```python
from build123d import *

# Parameters (mm, degrees)
SKETCH1_R             = 1.5500000000000012
BOSS_EXTRUDE1_DEPTH   = 1.5
SKETCH1_W             = 4.999999999999998
SKETCH1_H             = 10.5
BOSS_EXTRUDE1_2_DEPTH = 1.5
BOSS_EXTRUDE2_REACH   = 28.292
SKETCH2_R             = 2.500000000000001
SKETCH2_R_2           = 1.45
CUT_EXTRUDE1_DEPTH    = 25
FILLET1_R             = 2.5


with BuildPart() as part:
    # Sketch1 → Boss-Extrude1 (new, symmetric)
    with BuildSketch(Plane.XY):
        Polygon((-12.499999999999993, -2.4999999999999996), (-7.499999999999993, -2.5), (-7.499999999999993, 8), (-12.499999999999993, 8), align=None)
        with Locations((-9.999999999999995, 0)):
            Circle(SKETCH1_R, mode=Mode.SUBTRACT)
    extrude(amount=BOSS_EXTRUDE1_DEPTH, both=True)


with BuildPart() as body_2:
    # Sketch1 → Boss-Extrude1 2 (new, symmetric)
    with BuildSketch(Plane.XY):
        with Locations((10.000000000000007, 2.75)):
            Rectangle(SKETCH1_W, SKETCH1_H)
        with Locations((10.000000000000009, 2.45e-15)):
            Circle(SKETCH1_R, mode=Mode.SUBTRACT)
    extrude(amount=BOSS_EXTRUDE1_2_DEPTH, both=True)

    # Boss-Extrude2: up to this face of the body (flat: up to its plane)
    boss_extrude2_end = Plane(body_2.part.faces().sort_by_distance((12.5, 2.75, 0))[0])
    # Sketch2 → Boss-Extrude2 (add, up to the picked face)
    with BuildSketch(Plane.ZY.offset(12.499999999999993), mode=Mode.PRIVATE) as boss_extrude2_sk1:
        with Locations(Location((0, 8, 0), (0, 0, 306.869897646))):
            Circle(SKETCH2_R)
        with Locations((0, 8)):
            Circle(SKETCH2_R_2, mode=Mode.SUBTRACT)
    boss_extrude2_tool1 = split(extrude(boss_extrude2_sk1.sketch, amount=-BOSS_EXTRUDE2_REACH, mode=Mode.PRIVATE), bisect_by=boss_extrude2_end, keep=Keep.BOTH, mode=Mode.PRIVATE)

    add(part.part)  # Boss-Extrude2 merges part
    add(boss_extrude2_tool1.solids().sort_by(Axis((-12.5, 9.943431, -1.457574), (1, 0, 0)))[0])

    # Sketch2<2> → Cut-Extrude1 (cut)
    with BuildSketch(Plane.ZY.offset(12.499999999999993)):
        with BuildLine():
            Line((-1.4500000000000002, 8), (1.45, 8))
            ThreePointArc((1.45, 8), (9e-17, 9.45), (-1.45, 8))
        make_face()
        with BuildLine():
            ThreePointArc((-1.45, 8), (-2.7e-16, 6.55), (1.45, 8))
            Line((1.45, 8), (-1.4500000000000002, 8))
        make_face()
    extrude(amount=-CUT_EXTRUDE1_DEPTH, mode=Mode.SUBTRACT)

    # Fillet1
    fillet1_edges = [body_2.edges().sort_by_distance(p)[0] for p in [
        (7.500000000000007, -2.5, 0),
        (-7.499999999999993, -2.5, 0),
        (-12.499999999999993, -2.4999999999999996, 0),
        (12.500000000000007, -2.5, 0),
    ]]
    fillet(fillet1_edges, radius=FILLET1_R - 0.0001)  # a hair under: the kernel refuses the full size


solid = body_2.part
```
Check sheet for the modelled part. Datum: model origin and axes. Units: mm. A direction names the side the tool comes from. Give positions to 0.01 mm unless a question says otherwise; leave off trailing zeros. Order: outer loops, then holes, each group sorted by start corner. A loop starts at its lowest first (then second) coordinate and runs counter-clockwise, first axis right, second up. Notation, with made-up numbers: M 31.5,-5.75 L 49.5,-5.75 A29 cw 49.5,15.25 Z; hole C -21,18.5 d5. An arc over 180 degrees is marked long. Answer in a Markdown table with one row per item.
1) Cross-section at C-C, the plane x = -9.25. Enter the section's corners in (y, z), plus the area to 3 significant figures.
Filled sheet:
| item | result |
|---|---|
| outline | M -2.38,-1.5 L -1.36,-1.5 L -1.36,1.5 L -2.38,1.5 Z; M 1.36,-1.5 L 6,-1.5 A2.5 ccw long 6,1.5 L 1.36,1.5 Z; hole C 8,0 d2.9 |
| area | 29.0 mm2 |
2) Access from +Z, -Z, +X, -X, +Y, -Y to the whole of each face (thin tool, end or side, straight path). Record for faces 1 (the cylindrical face through (-0.175, 10.488, 0.246)), 2 (the cylindrical face through (8.213, -1.748, 0.021)), 3 (the flat face through (10, 3, -1.5)), 4 (the cylindrical face through (-11.14, 1.05, -0.02)), 5 (the flat face through (10, 3, 1.5)).
Filled sheet:
| item | result |
|---|---|
| face 1 | none |
| face 2 | +Z, -Z, -Y |
| face 3 | -Z, +X, -X, -Y |
| face 4 | +Z, -Z |
| face 5 | +Z, +X, -X, -Y |
3) Thickness scan on L1, parallel to Z at x = -1.5, y = 8; L2, parallel to Y at x = 10, z = -0.85; L3, parallel to Y at x = 11, z = -0.5. Record the ranges inside material, lowest first. Write a range as [from, to].
Filled sheet:
| item | result |
|---|---|
| L1 | z = [-2.5, -1.45], [1.45, 2.5] |
| L2 | y = [-2.5, -1.55], [1.55, 6.83], [9.17, 10.35] |
| L3 | y = [-2.29, -1.18], [1.18, 6.64], [9.36, 10.45] |
4) Gauge pin test, flat ends, axial feed: P1, Ø2.5, axis at y = 8, z = 0, coming from the +X side; P2, Ø4, axis at x = 10, y = 1.5, coming from the +Z side; P3, Ø6, axis at x = -9, y = 4, coming from the +Z side; P4, Ø4, axis at x = -0.5, y = 5.5, coming from the -Z side. Record the tip position at first contact, or that the pin passes through.
Filled sheet:
| item | result |
|---|---|
| P1 | passes through |
| P2 | stops at z = 1.5 |
| P3 | stops at z = 2.29 |
| P4 | stops at z = -2.45 |
5) Release check for a two-part mould opening along X. For faces 6 (the flat face through (-12.5, 5, 0)), 7 (the flat face through (-10, 3, 1.5)), 8 (the cylindrical face through (-8.213, -1.748, 0.021)), 9 (the flat face through (12.5, 5, 0)) record: +X half, -X half, draft (parallel to the pull), parting line (faces both ways), or undercut.
Filled sheet:
| item | result |
|---|---|
| face 6 | -X half |
| face 7 | draft |
| face 8 | undercut |
| face 9 | +X half |
6) Cross-section at A-A, the plane z = 0. Count the separate pieces of the cut face and the enclosed holes in it, plus the area to 3 significant figures.
Filled sheet:
| item | result |
|---|---|
| separate pieces | 2 |
| enclosed holes | 2 |
| area | 112 mm2 |
7) Cross-section at B-B, the plane y = 8. Enter the section's corners in (x, z), plus the area to 3 significant figures.
Filled sheet:
| item | result |
|---|---|
| outline | M -12.5,-2.5 L 12.5,-2.5 L 12.5,-1.45 L -12.5,-1.45 Z; M -12.5,1.45 L 12.5,1.45 L 12.5,2.5 L -12.5,2.5 Z |
| area | 52.5 mm2 |
